For this review, take the finished solid that the model builds, in its own axes (mm). Face numbers are marked on the shaded views. A direction names the side the tool comes from. Round coordinates to 2 decimals unless told otherwise and drop trailing zeros. Write each loop counter-clockwise with the first axis right and the second up, starting at its lowest first coordinate (ties: lowest second). Pieces come first, ordered by that corner, then holes. Notation, with made-up numbers: M -16,-14 L 14,-14 A24 cw 14,9 Z; hole C 47,-36.75 d5. An arc over 180 degrees is marked long. Answer in a Markdown table with one row per item.
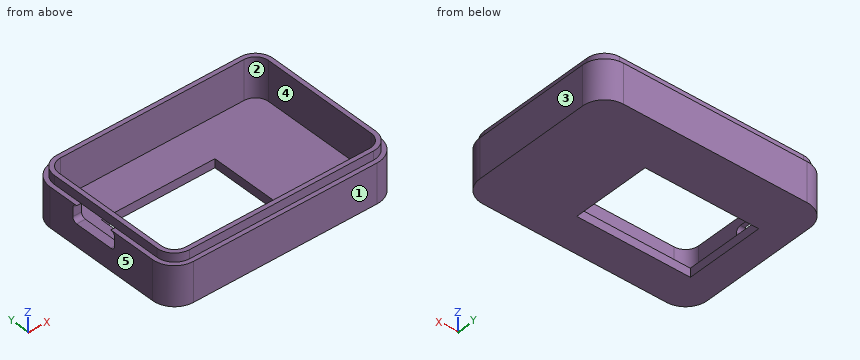
```python
from build123d import *

# Parameters (mm, degrees)
BOSS_EXTRU_1_DEPTH      = 11
COQUE5_T                = -2
ESQUISSE5_W             = 26
ESQUISSE5_H             = 18
ENL_V_MAT_EXTRU_4_DEPTH = 65.451532177
ESQUISSE6_OUTSIDE_W     = 66.952
ESQUISSE6_OUTSIDE_H     = 51.952
ENL_V_MAT_EXTRU_5_DEPTH = 2
ENL_V_MAT_EXTRU_6_DEPTH = 10


with BuildPart() as part:
    # Esquisse1 → Boss.-Extru.1 (new body)
    with BuildSketch(Plane.XY):
        with BuildLine():
            Line((5, 0), (47, 0))
            ThreePointArc((47, 0), (50.535533906, 1.464466094), (52, 5))
            Line((52, 5), (52, 32))
            ThreePointArc((52, 32), (50.535533906, 35.535533906), (47, 37))
            Line((47, 37), (5, 37))
            ThreePointArc((5, 37), (1.464466094, 35.535533906), (0, 32))
            Line((0, 32), (0, 5))
            ThreePointArc((0, 5), (1.464466094, 1.464466094), (5, 0))
        make_face()
    extrude(amount=BOSS_EXTRU_1_DEPTH)

    # Coque5
    coque5_openings = [part.faces().sort_by_distance(p)[0] for p in [
        (26, 18.5, 11),
    ]]
    offset(amount=COQUE5_T, openings=coque5_openings, kind=Kind.INTERSECTION)

    # Esquisse5 → Enlèv. mat.-Extru.4 (cut, through all)
    with BuildSketch(Plane.XY.offset(2)):
        with Locations((19.5, 17)):
            Rectangle(ESQUISSE5_W, ESQUISSE5_H)
    extrude(amount=-ENL_V_MAT_EXTRU_4_DEPTH, mode=Mode.SUBTRACT)

    # Esquisse6 outside → Enlèv. mat.-Extru.5 (cut)
    with BuildSketch(Plane.XY.offset(11)):
        with Locations((26, 18.5)):
            Rectangle(ESQUISSE6_OUTSIDE_W, ESQUISSE6_OUTSIDE_H)
        with BuildLine():
            Line((47, 36), (5, 36))
            ThreePointArc((5, 36), (2.171572875, 34.828427125), (1, 32))
            Line((1, 32), (1, 5))
            ThreePointArc((1, 5), (2.171572875, 2.171572875), (5, 1))
            Line((5, 1), (47, 1))
            ThreePointArc((47, 1), (49.828427125, 2.171572875), (51, 5))
            Line((51, 5), (51, 32))
            ThreePointArc((51, 32), (49.828427125, 34.828427125), (47, 36))
        make_face(mode=Mode.SUBTRACT)
    extrude(amount=-ENL_V_MAT_EXTRU_5_DEPTH, mode=Mode.SUBTRACT)

    # Esquisse7 → Enlèv. mat.-Extru.6 (cut)
    with BuildSketch(Plane.ZY):
        with BuildLine():
            Line((6, 26), (8, 26))
            ThreePointArc((8, 26), (8.707106781, 25.707106781), (9, 25))
            Line((9, 25), (9, 16))
            ThreePointArc((9, 16), (8.707106781, 15.292893219), (8, 15))
            Line((8, 15), (6, 15))
            ThreePointArc((6, 15), (5.292893219, 15.292893219), (5, 16))
            Line((5, 16), (5, 25))
            ThreePointArc((5, 25), (5.292893219, 25.707106781), (6, 26))
        make_face()
    extrude(amount=-ENL_V_MAT_EXTRU_6_DEPTH, mode=Mode.SUBTRACT)


solid = part.part
```
Q1. Take a section at D-D (y = 13). State the section outline as (x, z) points, then the cut area to 3 significant figures.
Found:
| item | result |
|---|---|
| outline | M 0,0 L 6.5,0 L 6.5,2 L 2,2 L 2,11 L 1,11 L 1,9 L 0,9 Z; M 32.5,0 L 52,0 L 52,9 L 51,9 L 51,11 L 50,11 L 50,2 L 32.5,2 Z |
| area | 84.0 mm² |
Q2. Take a section at C-C (x = 22.5). State the section outline as (y, z) points, then the cut area to 3 significant figures.
Found:
| item | result |
|---|---|
| outline | M 0,0 L 8,0 L 8,2 L 2,2 L 2,11 L 1,11 L 1,9 L 0,9 Z; M 26,0 L 37,0 L 37,9 L 36,9 L 36,11 L 35,11 L 35,2 L 26,2 Z |
| area | 70.0 mm² |
Q3. Mouldability with a two-part tool opening along Y and no side actions: class the marked faces 1, 2 and 3 as +Y half, -Y half, draft (parallel to the pull), parting line (faces both ways), or undercut.
Found:
| item | result |
|---|---|
| face 1 | -Y half |
| face 2 | undercut |
| face 3 | draft |
Q4. Take a section at A-A (y = 19). State the section outline as (x, z) points, then the cut area to 3 significant figures.
Found:
| item | result |
|---|---|
| outline | M 0,0 L 6.5,0 L 6.5,2 L 2,2 L 2,5 L 0,5 Z; M 1,9 L 2,9 L 2,11 L 1,11 Z; M 32.5,0 L 52,0 L 52,9 L 51,9 L 51,11 L 50,11 L 50,2 L 32.5,2 Z |
| area | 76.0 mm² |
Q5. Machinability: for the marked faces 4 and 5, which of the approach directions +Z, -Z, +X, -X, +Y, -Y give a long, thin tool a straight path to every point of the face, cutting with its end or side? Answer none if there is none.
Found:
| item | result |
|---|---|
| face 4 | +Z |
| face 5 | +Z, -Z, -X, +Y, -Y |
Q6. Insertion check: P1, Ø1.5, axis at x = 37.5, y = 27.5, coming from the +Z side; P2, Ø2, axis at y = 14, z = 10.5, coming from the +X side; P3, Ø0.6, axis at x = 21.5, z = 10, coming from the -Y side. Each pin has a flat end and moves straight along its axis. Give the tip position at first contact, or say it passes through.
Found:
| item | result |
|---|---|
| P1 | z = 2 |
| P2 | x = 51 |
| P3 | y = 1 |
Q7. Take a section at B-B (z = 4.25). State the section outline as (x, y) points.
Found:
| item | result |
|---|---|
| outline | M 0,5 A5 ccw 5,0 L 47,0 A5 ccw 52,5 L 52,32 A5 ccw 47,37 L 5,37 A5 ccw 0,32 Z; hole M 2,5 A3 ccw 5,2 L 47,2 A3 ccw 50,5 L 50,32 A3 ccw 47,35 L 5,35 A3 ccw 2,32 Z |
Q8. For probe 1 along Y at (x, z) = (28, 3); probe 2 along Y at (x, z) = (13, 9.5); probe 3 along X at (y, z) = (21, 10.25), list the stretches that pass through material, from the lowest coordinate up.
Found:
| item | result |
|---|---|
| probe 1 | 0 to 2, 35 to 37 |
| probe 2 | 1 to 2, 35 to 36 |
| probe 3 | 1 to 2, 50 to 51 |
